from build123d import *

# Parameters (mm, degrees)
FILLET1_R          = 0.1
SKETCH2_R          = 2
CUT_EXTRUDE1_DEPTH = 0.5
CUT_EXTRUDE2_REACH = 7.5
SKETCH3_R          = 1.5


with BuildPart() as part:
    # Sketch1 → Revolve1 (revolve)
    with BuildSketch(Plane.XY):
        Polygon((0, 0), (-4.054195804, 0), (-4.054195804, -1.5), (-1.554195804, -1.5), (-1.554195804, -3), (5.445804196, -3), (5.445804196, -1.5), (7.945804196, -1.5), (7.945804196, 0), align=None)
    revolve(axis=Axis((7.945804196, 0, 0), (-1, 0, 0)))

    # Fillet1
    fillet1_edges = [part.edges().sort_by_distance(p)[0] for p in [
        (7.945804196, 1.5, 0),
        (5.445804196, 3, 0),
        (-1.554195804, 3, 0),
        (-4.054195804, 1.5, 0),
    ]]
    fillet(fillet1_edges, radius=FILLET1_R)

    # Sketch2 → Cut-Extrude1 (cut)
    with BuildSketch(Plane.XY.offset(3)):
        with Locations((1.945804196, 0)):
            Circle(SKETCH2_R)
    extrude(amount=-CUT_EXTRUDE1_DEPTH, mode=Mode.SUBTRACT)

    # Sketch3 → Cut-Extrude2 (cut, up to next)
    with BuildSketch(Plane.XY.offset(2.5), mode=Mode.PRIVATE) as cut_extrude2_sk1:
        with Locations((1.945804196, 0)):
            Circle(SKETCH3_R)
    cut_extrude2_tool1 = extrude(cut_extrude2_sk1.sketch, amount=-CUT_EXTRUDE2_REACH, mode=Mode.PRIVATE) & part.part
    add(cut_extrude2_tool1.solids().sort_by_distance((1.945804, 0, 2.5))[0], mode=Mode.SUBTRACT)


solid = part.part
Source: CAD feature listing. Evaluate the final solid. Frame: model axes, mm. A direction names the side the tool comes from. Give positions to 0.01 mm unless a question says otherwise; leave off trailing zeros. Write each loop counter-clockwise with the first axis right and the second up, starting at its lowest first coordinate (ties: lowest second). Pieces come first, ordered by that corner, then holes. Notation, with made-up numbers: M 19.25,-30 L 30.25,-30 A6 cw 30.25,-23 Z; hole C -31.5,34.5 d3. An arc over 180 degrees is marked long. Return JSON: item names as keys, results as strings. Group by question number.
1) Pull-direction query (X, two-part tool) for faces 5 (the face through (-2.74, 1.5, 0.07)), 6 (the face through (7.946, 0, 0)), 7 (the face through (-0.054, 0.027, 2.698)); classes: pulls with the +X half, pulls with the -X half, needs draft (parallel to the pull), parting line crosses it, or undercut.
2) Cut plane A-A, the plane z = 0. Output: boundary loops of the cut face in (x, y).
3) Material intervals for line 1 along X through (y, z) = (0, -1); line 2 along X through (y, z) = (0, -1.6); line 3 along X through (y, z) = (-2, -0.5), sorted ascending. Write a range as [from, to].
4) Set-up query: faces 1 (the face through (3.946, -0.027, 2.698)), 2 (the face through (-1.554, 1.2, -1.2)), 3 (the face through (5.446, -1.2, -1.2)), 4 (the face through (2, 2.4, -1.8)). Return all of +Z, -Z, +X, -X, +Y, -Y with unobstructed straight access to the full face (end or side cutting, diameter ignored); none if empty.
5) Pin query (flat end, axial travel): P1, Ø1, axis at x = 2.5, y = 0, coming from the +Z side; P2, Ø1, axis at y = 0.5, z = -1.5, coming from the -X side; P3, Ø2, axis at y = -2.5, z = -2, coming from the +X side; P4, Ø3.5, axis at x = 1.95, y = 0, coming from the +Z side. Return the tip coordinate at first contact, or that it passes through.
6) Cut plane B-B, the plane x = -2.25. Output: boundary loops of the cut face in (y, z).
Recorded:
{
 "1": {"face 5": "needs draft", "face 6": "pulls with the +X half", "face 7": "undercut"},
 "2": {"outline": "M -4.05,-1.4 A0.1 ccw -3.95,-1.5 L -1.55,-1.5 L -1.55,-2.9 A0.1 ccw -1.45,-3 L 5.35,-3 A0.1 ccw 5.45,-2.9 L 5.45,-1.5 L 7.85,-1.5 A0.1 ccw 7.95,-1.4 L 7.95,1.4 A0.1 ccw 7.85,1.5 L 5.45,1.5 L 5.45,2.9 A0.1 ccw 5.35,3 L -1.45,3 A0.1 ccw -1.55,2.9 L -1.55,1.5 L -3.95,1.5 A0.1 ccw -4.05,1.4 Z; hole C 1.95,0 d3"},
 "3": {"line 1": "x = [-4.05, 0.45], [3.45, 7.95]", "line 2": "x = [-1.55, 0.45], [3.45, 5.45]", "line 3": "x = [-1.55, 5.45]"},
 "4": {"face 1": "+Z", "face 2": "-X", "face 3": "+X", "face 4": "+X, -X"},
 "5": {"P1": "passes through", "P2": "stops at x = -4.05", "P3": "stops at x = 5.45", "P4": "stops at z = 2.5"},
 "6": {"outline": "C 0,0 d3"}
}
